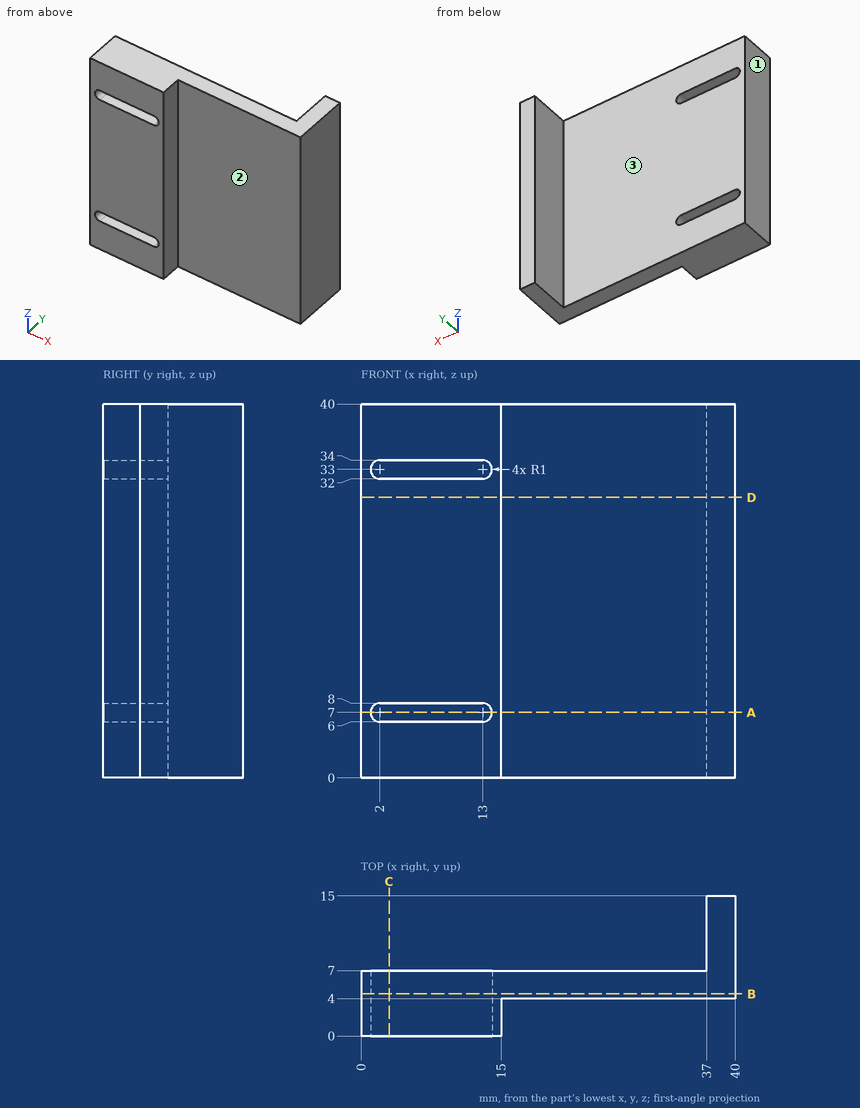
Part print with two shaded views. Sizes in mm from the minimum x, y, z corner. A direction names the side the tool comes from. Round coordinates to 2 decimals unless told otherwise and drop trailing zeros. Loops run counter-clockwise (first coordinate to the right, second up) from the corner with the lowest first, then second, coordinate; pieces in that order, holes last. Notation, with made-up numbers: M 8.25,89 L 38.25,89 A23 ccw 38.25,98 Z; hole C -12.75,-24.75 d1. An arc over 180 degrees is marked long. Return JSON: item names as keys, results as strings. Group by question number.
(1) Saw through at A-A, the plane z = 7. List the corners of the cut face in (x, y).
(2) Tool access for the marked faces 1, 2 and 3: list every direction of +Z, -Z, +X, -X, +Y, -Y with a clear straight run to the whole face (end or side of a thin tool).
(3) Saw through at D-D, the plane z = 30. List the corners of the cut face in (x, y), and give its area (3 significant figures).
(4) Wall check: probe 1 along Z at (x, y) = (2.5, 6); probe 2 along X at (y, z) = (13.5, 11); probe 3 along Y at (x, z) = (16, 10). Give the ranges that are in metal, low to high. Write a range as [from, to].
(5) Saw through at C-C, the plane x = 3. List the corners of the cut face in (y, z), and give its area (3 significant figures).
(6) Saw through at B-B, the plane y = 4.5. List the corners of the cut face in (x, z), and give its area (3 significant figures).
(7) Drop flat-ended pins along their axis: P1, Ø6, axis at x = 19, z = 21, coming from the +Y side; P2, Ø1.2, axis at y = 2.5, z = 28.5, coming from the +X side; P3, Ø7.5, axis at x = 26.5, z = 26, coming from the -Y side. Give the stop position or say it passes through.
Answer list:
{
 "1": {"outline": "M 0,0 L 1,0 L 1,7 L 0,7 Z; M 14,0 L 15,0 L 15,4 L 40,4 L 40,15 L 37,15 L 37,7 L 14,7 Z"},
 "2": {"face 1": "+Z, -Z, -X, +Y, -Y", "face 2": "+Z, -Z, +X, -Y", "face 3": "+Z, -Z, -X, +Y"},
 "3": {"outline": "M 0,0 L 15,0 L 15,4 L 40,4 L 40,15 L 37,15 L 37,7 L 0,7 Z", "area": "204 mm2"},
 "4": {"probe 1": "[0, 6], [8, 32], [34, 40]", "probe 2": "[37, 40]", "probe 3": "[4, 7]"},
 "5": {"outline": "M 0,0 L 7,0 L 7,6 L 0,6 Z; M 0,8 L 7,8 L 7,32 L 0,32 Z; M 0,34 L 7,34 L 7,40 L 0,40 Z", "area": "252 mm2"},
 "6": {"outline": "M 0,0 L 40,0 L 40,40 L 0,40 Z; hole M 2,6 L 13,6 A1 ccw 13,8 L 2,8 A1 ccw Z; hole M 2,32 L 13,32 A1 ccw 13,34 L 2,34 A1 ccw Z", "area": "1,550 mm2"},
 "7": {"P1": "y = 7", "P2": "x = 15", "P3": "y = 4"}
}
